Input: part model. Units: mm. Frame: model coordinates. Face numbers are marked on the shaded views. A direction names the side the tool comes from. Coordinates: 2 decimals unless noted, no trailing zeros. Loops run counter-clockwise (first coordinate to the right, second up) from the corner with the lowest first, then second, coordinate; pieces in that order, holes last. Notation, with made-up numbers: (87.25, -40) -> (141.25, -40) arc R31 ccw to (141.25, -12) -> close; hole circle Ø3 at (69.25, -14.5). An arc over 180 degrees is marked (long way). Put each result on its own line as item: value. Start each with the question number.
1) Cut plane A-A (z = 0). Return the cut outline in (x, y).
2) Cut plane C-C (x = 100.5). Return the cut outline in (y, z), plus the area to 3 significant figures.
3) Set-up query: the marked faces 1, 2 and 3. Return all of +Z, -Z, +X, -X, +Y, -Y with unobstructed straight access to the full face (end or side cutting, diameter ignored); none if empty.
4) Cut plane D-D (x = 35). Return the cut outline in (y, z).
5) Contact query for flat-ended pins moving along their axis: P1, Ø6, axis at x = 73, z = 5, coming from the -Y side; P2, Ø1.5, axis at y = -8, z = 9.5, coming from the +X side; P3, Ø12, axis at x = 60, y = -4.5, coming from the -Z side; P4, Ø1, axis at x = 97.5, z = -11, coming from the -Y side. Output: stop coordinate, or through.
6) Material intervals for L1, parallel to X at y = -12, z = -7.5; L2, parallel to Z at x = 54, y = -0.5; L3, parallel to X at y = 7.25, z = 7.75, sorted ascending.
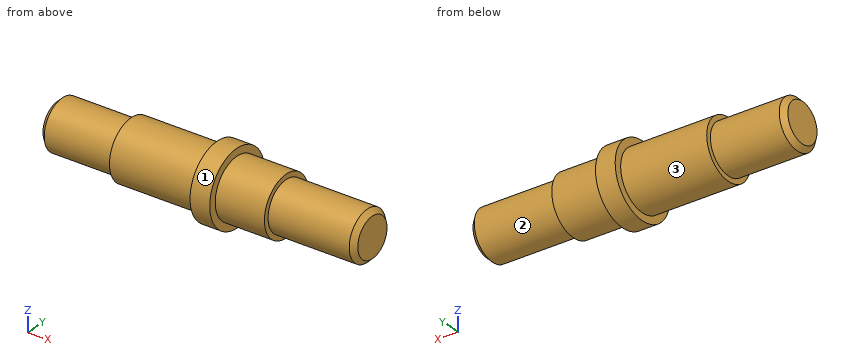
from build123d import *

# Parameters (mm, degrees)
ZKOSEN_1_SIZE = 2


with BuildPart() as part:
    # Skica1 → Rotovat1 (revolve)
    with BuildSketch(Plane.XY):
        Polygon((0, 0), (0, 10), (30, 10), (30, 12), (65, 12), (65, 15), (73, 15), (73, 12), (93, 12), (93, 10), (128, 10), (128, 0), align=None)
    revolve(axis=Axis((128, 0, 0), (-1, 0, 0)))

    # Zkosení1
    zkosen_1_edges = [part.edges().sort_by_distance(p)[0] for p in [
        (0, -10, 0),
        (128, -10, 0),
    ]]
    chamfer(zkosen_1_edges, length=ZKOSEN_1_SIZE)


solid = part.part
Results found:
1. outline: (0, -8) -> (2, -10) -> (30, -10) -> (30, -12) -> (65, -12) -> (65, -15) -> (73, -15) -> (73, -12) -> (93, -12) -> (93, -10) -> (126, -10) -> (128, -8) -> (128, 8) -> (126, 10) -> (93, 10) -> (93, 12) -> (73, 12) -> (73, 15) -> (65, 15) -> (65, 12) -> (30, 12) -> (30, 10) -> (2, 10) -> (0, 8) -> close
2. outline: circle Ø20 at (0, 0)
2. area: 314 mm2
3. face 1: +X, -X
3. face 2: +X
3. face 3: -X
4. outline: circle Ø24 at (0, 0)
5. P1: stops at y = -14.87
5. P2: stops at x = 93
5. P3: stops at z = -14.95
5. P4: passes through
6. L1: x = 65 to 73
6. L2: z = -11.99 to 11.99
6. L3: x = 30 to 93
